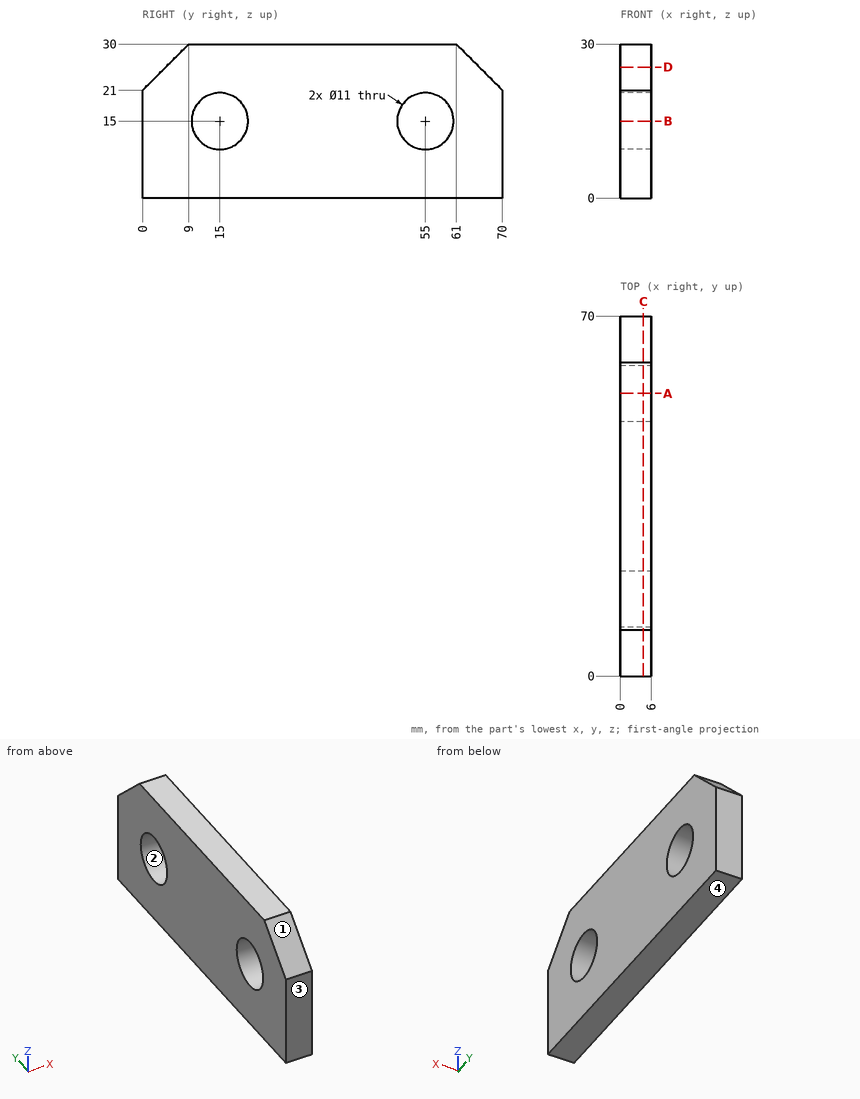
The drawing under review shows one solid part. Ordinate dimensions are in mm from its lowest x, y, z. Coordinates: 2 decimals unless noted, no trailing zeros. Write each loop counter-clockwise with the first axis right and the second up, starting at its lowest first coordinate (ties: lowest second). Pieces come first, ordered by that corner, then holes. Notation, with made-up numbers: (68, -30) - (113, -30) arc R23 cw to (113, -8) - close; hole circle Ø2 at (37.25, -14). An arc over 180 degrees is marked (long way). Put each result on its own line as item: value.
1. Add section B-B, the plane z = 15. Give the boundary of the cut face in (x, y), then the cut area to 3 significant figures.
Values found:
outline: (0, 0) - (6, 0) - (6, 9.5) - (0, 9.5) - close; (0, 20.5) - (6, 20.5) - (6, 49.5) - (0, 49.5) - close; (0, 60.5) - (6, 60.5) - (6, 70) - (0, 70) - close
area: 288 mm²
2. Add section A-A, the plane y = 55. Give the boundary of the cut face in (x, z), then the cut area to 3 significant figures.
Values found:
outline: (0, 0) - (6, 0) - (6, 9.5) - (0, 9.5) - close; (0, 20.5) - (6, 20.5) - (6, 30) - (0, 30) - close
area: 114 mm²
3. Add section C-C, the plane x = 4.45. Give the boundary of the cut face in (y, z), then the cut area to 3 significant figures.
Values found:
outline: (0, 0) - (70, 0) - (70, 21) - (61, 30) - (9, 30) - (0, 21) - close; hole circle Ø11 at (15, 15); hole circle Ø11 at (55, 15)
area: 1,830 mm²
4. Mouldability with a two-part tool opening along Z and no side actions: class the marked faces 1, 2, 3 and 4 as released by +Z, released by -Z, zero draft, split by the parting line, or undercut.
Values found:
face 1: released by +Z
face 2: undercut
face 3: zero draft
face 4: released by -Z
5. Add section D-D, the plane z = 25.5. Give the boundary of the cut face in (x, y), then the cut area to 3 significant figures.
Values found:
outline: (0, 4.5) - (6, 4.5) - (6, 65.5) - (0, 65.5) - close
area: 366 mm²
6. For pin 1 (1.5 mm diameter, centred on x = 3.5, z = 20.5, fed in from -Y), flat-tipped, find the tip position at first contact; note if it passes through.
Values found:
pin 1: y = 0
7. Wall thickness on probe 1 along Z at (x, y) = (1.4, 55); probe 2 along Y at (x, z) = (1.45, 10.75); probe 3 along Z at (x, y) = (1.65, 12): over which ranges is each line inside the solid? List them lowest first.
Values found:
probe 1: 0 to 9.5, 20.5 to 30
probe 2: 0 to 11.51, 18.49 to 51.51, 58.49 to 70
probe 3: 0 to 10.39, 19.61 to 30
